Source: three-view drawing plus pictorial views. Frame: mm from the lowest corner of the part. Give positions to 0.01 mm unless a question says otherwise; leave off trailing zeros. Loops run counter-clockwise (first coordinate to the right, second up) from the corner with the lowest first, then second, coordinate; pieces in that order, holes last. Notation, with made-up numbers: (-29.5, 72.5) - (29.5, 72.5) arc R36 ccw to (29.5, 109.5) - close; hole circle Ø11 at (-32, 43). An arc over 180 degrees is marked (long way). Write each question's results on one line, items separated by ' | '. Start each with the question number.
(1) Material intervals for line 1 along Y through (x, z) = (228, 4.75); line 2 along Y through (x, z) = (187.5, 15.25); line 3 along X through (y, z) = (444, 1.25), sorted ascending. Write a range as [from, to].
(2) Cut plane B-B on x = 172.85. Return the cut outline in (y, z).
(3) Cut plane A-A on y = 481. Return the cut outline in (x, z).
(4) Cut plane D-D on y = 117. Return the cut outline in (x, z), then the cut area to 3 significant figures.
(5) Cut plane C-C on z = 5.25. Give the number of separate pieces and of enclosed holes in the cut face, then the cut area to 3 significant figures.
(6) Contact query for flat-ended pins moving along their axis: pin 1 (1 mm diameter, centred on x = 167.5, z = 2, fed in from -Y); pin 2 (5 mm diameter, centred on x = 93.88, y = 310.91, fed in from +Z). Output: stop coordinate, or through.
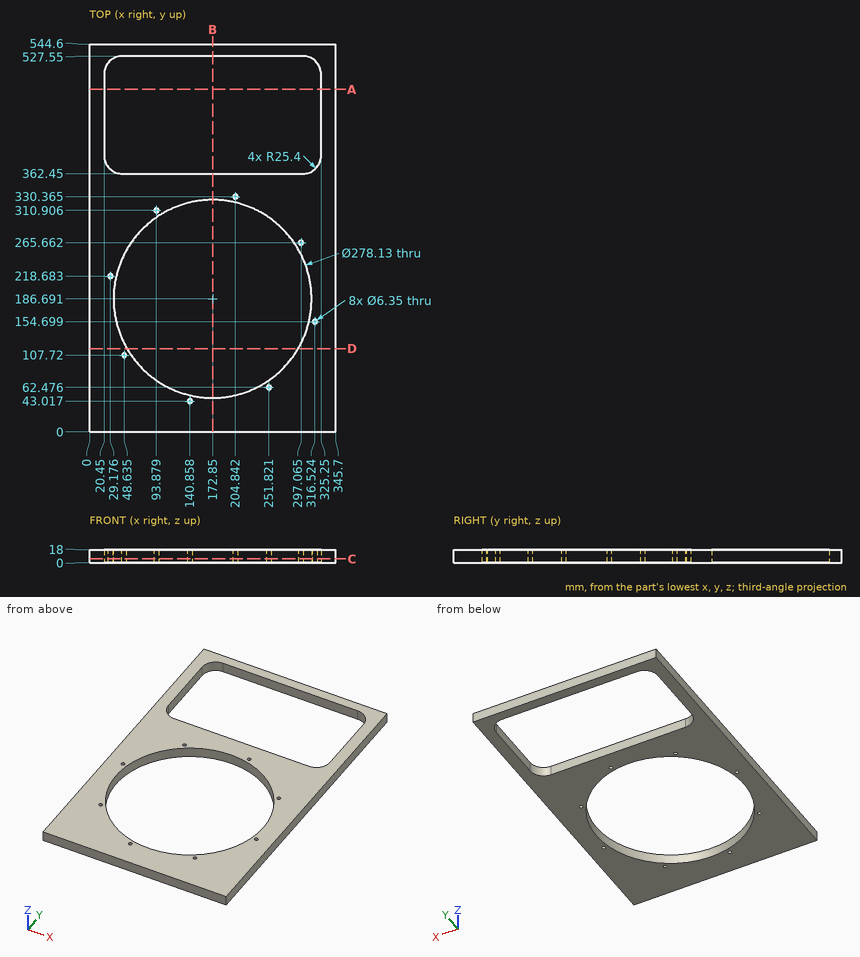
Ans:
1) line 1: [0, 59.03], [314.35, 362.45], [527.55, 544.6] | line 2: [0, 48.4], [324.98, 362.45], [527.55, 544.6] | line 3: [0, 20.45], [325.25, 345.7]
2) outline: (0, 0) - (47.63, 0) - (47.63, 18) - (0, 18) - close; (325.76, 0) - (362.45, 0) - (362.45, 18) - (325.76, 18) - close; (527.55, 0) - (544.6, 0) - (544.6, 18) - (527.55, 18) - close
3) outline: (0, 0) - (20.45, 0) - (20.45, 18) - (0, 18) - close; (325.25, 0) - (345.7, 0) - (345.7, 18) - (325.25, 18) - close
4) outline: (0, 0) - (52.51, 0) - (52.51, 18) - (0, 18) - close; (293.19, 0) - (345.7, 0) - (345.7, 18) - (293.19, 18) - close | area: 1,890 mm^2
5) separate pieces: 1 | enclosed holes: 10 | area: 77,500 mm^2
6) pin 1: y = 0 | pin 2: through
